Job drawing, mm, ordinate dimensions from the low corner. One solid piece. A direction names the side the tool comes from. Round coordinates to 2 decimals unless told otherwise and drop trailing zeros. Write each loop counter-clockwise with the first axis right and the second up, starting at its lowest first coordinate (ties: lowest second). Pieces come first, ordered by that corner, then holes.
1) Saw through at B-B (x = 70). Write the cut outline in (y, z), plus the area to 3 significant figures.
2) Saw through at C-C (x = 20). Write the cut outline in (y, z).
3) Flat gauge pins, fed straight in: pin 1 (13.5 mm diameter, centred on x = 20, y = 15, fed in from -Z); pin 2 (3 mm diameter, centred on y = 12.5, z = 97.5, fed in from -X). Where does each tip first touch, or does it go through?
4) Wall check: probe 1 along Z at (x, y) = (39, 17); probe 2 along Y at (x, z) = (70, 30.5); probe 3 along X at (y, z) = (18.25, 6). Give the ranges that are in metal, low to high.
5) Saw through at A-A (y = 15). Write the cut outline in (x, z).
6) Pull direction Y, two halves, no side cores. Call the marked faces 3, 4 and 5: +Y half, -Y half, draft (parallel to the pull), parting line (faces both ways), or undercut.
7) Which spindle directions (+Z, -Z, +X, -X, +Y, -Y) get a long thin tool onto all of the face, cutting with end or side? Do the marked faces 1 and 2. Say none if no direction does.
8) Saw through at D-D (z = 18). Write the cut outline in (x, y).
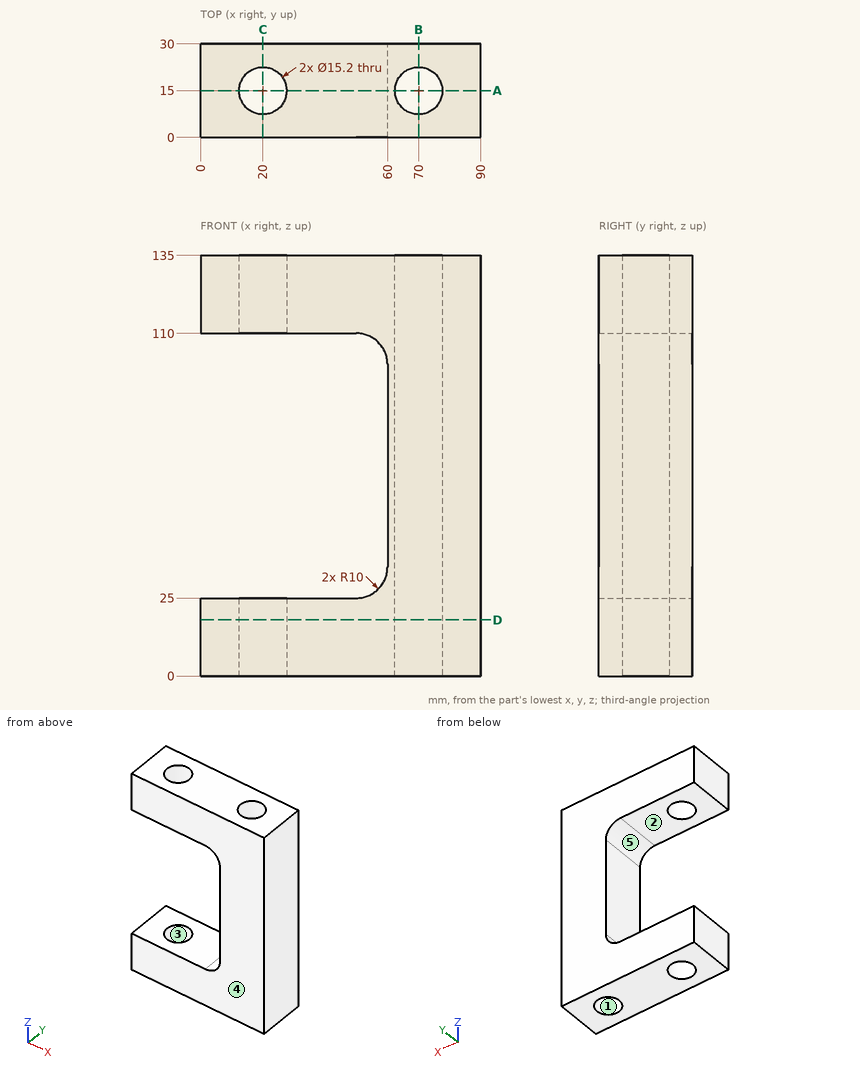
Evaluation:
1. outline: (0, 0) - (7.4, 0) - (7.4, 135) - (0, 135) - close; (22.6, 0) - (30, 0) - (30, 135) - (22.6, 135) - close
1. area: 2,000 mm2
2. outline: (0, 0) - (7.4, 0) - (7.4, 25) - (0, 25) - close; (0, 110) - (7.4, 110) - (7.4, 135) - (0, 135) - close; (22.6, 0) - (30, 0) - (30, 25) - (22.6, 25) - close; (22.6, 110) - (30, 110) - (30, 135) - (22.6, 135) - close
3. pin 1: passes through
3. pin 2: stops at x = 60
4. probe 1: z = 0 to 25, 110 to 135
4. probe 2: y = 0 to 7.4, 22.6 to 30
4. probe 3: x = 0 to 13.13, 26.87 to 63.13, 76.87 to 90
5. outline: (0, 0) - (12.4, 0) - (12.4, 25) - (0, 25) - close; (0, 110) - (12.4, 110) - (12.4, 135) - (0, 135) - close; (27.6, 0) - (62.4, 0) - (62.4, 135) - (27.6, 135) - (27.6, 110) - (50, 110) arc R10 cw to (60, 100) - (60, 35) arc R10 cw to (50, 25) - (27.6, 25) - close; (77.6, 0) - (90, 0) - (90, 135) - (77.6, 135) - close
6. face 3: undercut
6. face 4: -Y half
6. face 5: draft
7. face 1: +Z, -Z
7. face 2: -X, +Y, -Y
8. outline: (0, 0) - (90, 0) - (90, 30) - (0, 30) - close; hole circle Ø15.2 at (20, 15); hole circle Ø15.2 at (70, 15)
